Autodesk Inventor part; units mm, degrees
ref_plane "YZ Plane" through (0, 0, 0) normal (1, 0, 0) x (0, 1, 0)
ref_plane "XZ Plane" through (0, 0, 0) normal (0, 1, 0) x (-1, 0, 0)
ref_plane "XY Plane" through (0, 0, 0) normal (0, 0, 1) x (1, 0, 0)
sketch "Sketch1" plane through (0, 0, 0) normal (1, 0, 0) x (0, 1, 0)
  line L0 (-2.825, 8) -> (2.825, 8)
  line L1 (2.825, 8) -> (2.825, -8)
  line L2 (2.825, -8) -> (-2.825, -8)
  line L3 (-2.825, -8) -> (-2.825, 8)
  line L4 (-2.825, 8) -> (2.825, -8) construction
  line L5 (2.825, 8) -> (-2.825, -8) construction
  point P0 (0, 0)
  dimension "d0" = 5.65
  dimension "d1" = 16
extrude "Extrusion1" add sketch "Sketch1" along normal blind 1.53
sketch "Sketch2" plane through (1.53, 0, 0) normal (1, 0, 0) x (0, 0, -1)
  line L0 (8, 2.825) -> (-8, 2.825)
  line L1 (-6.1, -2.825) -> (6.1, -2.825)
  line L2 (6.1, -2.825) -> (6.1, 2.825) construction
  line L3 (6.1, 2.825) -> (-6.1, 2.825)
  line L4 (-6.1, 2.825) -> (-6.1, -2.825) construction
  line L5 (-6.1, -2.825) -> (6.1, 2.825) construction
  line L6 (6.1, -2.825) -> (-6.1, 2.825) construction
  point P0 (0, 0)
  point P1 (6.1, 0)
  point P2 (-6.1, 0)
  dimension "d4" = 12.2
hole "Hole1" at (1.53, 0, -6.1) at (1.53, 0, 6.1) direction (-1, 0, 0) diameter 2.6 end through all
chamfer "Chamfer1" distance 1.9 angle 45 4 edges at (0.765, 2.825, 8) (0.765, 2.825, -8) (0.765, -2.825, 8) (0.765, -2.825, -8)
sketch "Sketch3" plane through (1.53, 0, 0) normal (1, 0, 0) x (0, 0, -1)
  circle A0 centre (0, 0) radius 2.03
  dimension "d15" = 4.06
extrude "Extrusion2" add sketch "Sketch3" along normal blind 12.7
sketch "Sketch4" plane through (14.23, 0, 0) normal (1, 0, 0) x (0, 0, -1)
  circle A0 centre (0, 0) radius 0.6375
  dimension "d18" = 1.275
extrude "Extrusion3" add sketch "Sketch4" along normal blind 3.2
sketch "Sketch5" plane through (0, 0, 0) normal (-1, 0, 0) x (0, 0, 1)
  circle A0 centre (0, 0) radius 2
  dimension "d21" = 4
extrude "Extrusion4" add sketch "Sketch5" along normal blind 2
sketch "Sketch6" plane through (-2, 0, 0) normal (-1, 0, 0) x (0, 0, 1)
  circle A0 centre (0, 0) radius 3
  dimension "d24" = 6
extrude "Extrusion5" add sketch "Sketch6" along normal blind 6
thread "Thread1"
sketch "Sketch7" plane through (-8, 0, 0) normal (-1, 0, 0) x (0, 0, 1)
  circle A0 centre (0, 0) radius 0.6375
hole "Hole2" at (-8, 0, 0) direction (1, 0, 0) diameter 0.7294 depth 3.5 tip angle 118
sketch "Sketch8" plane through (-8, 0, 0) normal (-1, 0, 0) x (0, 0, 1)
  circle A0 centre (0, 0) radius 0.3647
  circle A1 centre (0, 0) radius 2.5
  dimension "d36" = 5
extrude "Extrusion6" cut sketch "Sketch8" against normal blind 2
properties part number "SMAPanel1" material "Brass, Soft Yellow"
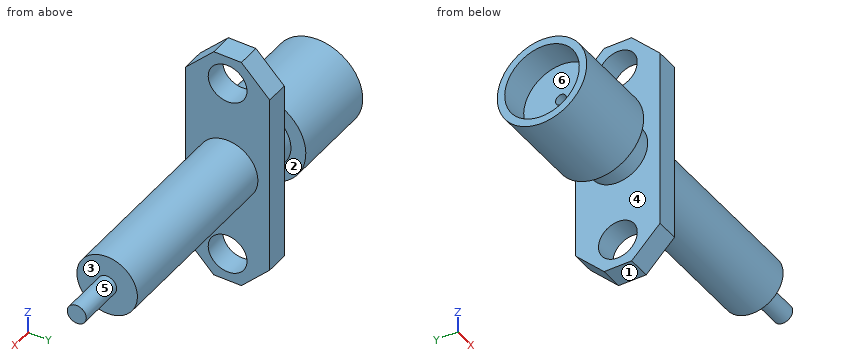
Read the model definition and answer for the solid it produces. Units are mm, in the model's axes. Face numbers are marked on the shaded views. A direction names the side the tool comes from. Give positions to 0.01 mm unless a question says otherwise; leave off trailing zeros. Order: outer loops, then holes, each group sorted by start corner. A loop starts at its lowest first (then second) coordinate and runs counter-clockwise, first axis right, second up. Notation, with made-up numbers: (57.25, -7) -> (86.25, -7) arc R28 ccw to (86.25, 31) -> close; hole circle Ø6 at (-23.75, -6.5). An arc over 180 degrees is marked (long way). One line per item, written item: value. Start each with the question number.
(1) Straight lines are drawn through the part: L1, parallel to Z at x = 1.1, y = 0; L2, parallel to X at y = -0.4, z = 2.75; L3, parallel to Y at x = -7.15, z = 0. For each, find the intervals that lie inside material, in ascending order.
(2) The part is cut by section D-D (z = 3.25). Determine the outline of the cut face in (x, y) (3 decimals).
(3) A tool of negligible diameter and unlimited length cuts with its end or side. For the marked faces 4, 5 and 6, from which of +Z, -Z, +X, -X, +Y, -Y can it reach the whole face along a straight path? Write none if from no direction.
(4) The part is cut by section A-A (z = -7). Determine the outline of the cut face in (x, y) (3 decimals).
(5) For a pull along X with two mould halves and no side action, classify the marked faces 1, 2 and 3 as released by +X, released by -X, zero draft, split by the parting line, or undercut.
(6) Flat-ended cylindrical pins translate along their axes: P1, Ø1.7, axis at x = 1, z = -1, coming from the +Y side (3 decimals); P2, Ø3, axis at y = 1, z = 0.5, coming from the +X side; P3, Ø3.5, axis at y = 0, z = 6.1, coming from the -X side; P4, Ø2, axis at x = -4, y = 1, coming from the -Z side. Find the tip coordinate at first contact, or state that the pin passes through.
(7) The part is cut by section C-C (x = 3.5). Determine the outline of the cut face in (y, z), and give its area (3 significant figures).
(8) The part is cut by section B-B (y = -1.6). Determine the outline of the cut face in (x, z) (3 decimals).
Taken from the geometry:
1. L1: -8 to -7.4, -4.8 to 4.8, 7.4 to 8
1. L2: -8 to -2, 0 to 1.53
1. L3: -3 to -2.5, 2.5 to 3
2. outline: (0, -2.825) -> (1.53, -2.825) -> (1.53, 2.825) -> (0, 2.825) -> close
3. face 4: none
3. face 5: +X
3. face 6: -X
4. outline: (0, -1.925) -> (1.53, -1.925) -> (1.53, -0.938) -> (0, -0.938) -> close; (0, 0.938) -> (1.53, 0.938) -> (1.53, 1.925) -> (0, 1.925) -> close
5. face 1: zero draft
5. face 2: undercut
5. face 3: released by +X
6. P1: y = 2.825
6. P2: x = 17.43
6. P3: x = 0
6. P4: z = -3
7. outline: circle Ø4.06 at (0, 0)
7. area: 12.9 mm^2
8. outline: (-8, -2.538) -> (-2, -2.538) -> (-2, -1.2) -> (0, -1.2) -> (0, -7.325) -> (1.53, -7.325) -> (1.53, -1.249) -> (14.23, -1.249) -> (14.23, 1.249) -> (1.53, 1.249) -> (1.53, 7.325) -> (0, 7.325) -> (0, 1.2) -> (-2, 1.2) -> (-2, 2.538) -> (-8, 2.538) -> (-8, 1.921) -> (-6, 1.921) -> (-6, -1.921) -> (-8, -1.921) -> close
